Could you check a few things on this model? Use its own coordinates, in mm. A direction names the side the tool comes from. Round coordinates to 2 decimals unless told otherwise and drop trailing zeros. Write each loop counter-clockwise with the first axis right and the second up, starting at its lowest first coordinate (ties: lowest second). Pieces come first, ordered by that corner, then holes. Notation, with made-up numbers: (17, 15.25) - (66, 15.25) arc R21 cw to (66, 30.25) - close; hole circle Ø2 at (-32, -35). An arc over 180 degrees is marked (long way). Put each result on its own line as item: value.
from build123d import *

# Parameters (mm, degrees)
CHAMFER_1_SIZE      = 0.5
SKETCH_2_R          = 1.65
CUT_EXTRUDE_1_DEPTH = 10
SKETCH_3_R          = 1.65
CUT_EXTRUDE_2_DEPTH = 10


with BuildPart() as part:
    # 草图1 → 旋转1 (revolve)
    with BuildSketch(Plane(origin=(0, 0, 0), x_dir=(1, 0, 0), z_dir=(0, 1, 0)), mode=Mode.PRIVATE) as revolve_1_sk:
        Polygon((25, 8), (0, 8), (0, 2.5), (12.5, 2.5), (12.5, 4), (25, 4), align=None)
    revolve(revolve_1_sk.sketch.rotate(Axis((-10.524691358, 0, 0), (1, 0, 0)), 180), axis=Axis((-10.524691358, 0, 0), (1, 0, 0)))

    # 倒角1
    chamfer_1_edges = [part.edges().sort_by_distance(p)[0] for p in [
        (25, 0, -4),
        (12.5, 0, -2.5),
        (0, 0, -2.5),
        (0, 0, -8),
        (25, 0, -8),
    ]]
    chamfer(chamfer_1_edges, length=CHAMFER_1_SIZE)

    # 草图2 → 切除-拉伸1 (cut)
    with BuildSketch(Plane(origin=(0, 0, 0), x_dir=(1, 0, 0), z_dir=(0, 1, 0))):
        with Locations(Location((5, 0, 0), (0, 0, 270))):
            Circle(SKETCH_2_R)
        with Locations(Location((20, 0, 0), (0, 0, 270))):
            Circle(SKETCH_2_R)
    extrude(amount=-CUT_EXTRUDE_1_DEPTH, mode=Mode.SUBTRACT)

    # 草图3 → 切除-拉伸2 (cut)
    with BuildSketch(Plane.XY):
        with Locations((5, 0)):
            Circle(SKETCH_3_R)
        with Locations((20, 0)):
            Circle(SKETCH_3_R)
    extrude(amount=-CUT_EXTRUDE_2_DEPTH, mode=Mode.SUBTRACT)


solid = part.part
(1) Imagine slicing it at C-C, the plane x = 20. List the corners of the cut face in (y, z) for me.
Values found:
outline: (-7.83, -1.65) arc R8 ccw to (-1.65, -7.83) - (-1.65, -3.64) arc R4 cw to (-3.64, -1.65) - close; (-7.83, 1.65) - (-3.64, 1.65) arc R4 cw (long way) to (1.65, -3.64) - (1.65, -7.83) arc R8 ccw (long way) to start
(2) I'm going to push flat-ended pins straight in: pin 1 (6 mm diameter, centred on x = 8.5, z = 5, fed in from -Y); pin 2 (1 mm diameter, centred on x = 3.5, y = -6, fed in from -Z); pin 3 (5 mm diameter, centred on x = 7.5, z = 6.5, fed in from -Y); pin 4 (4.5 mm diameter, centred on y = 0, z = 0, fed in from -X). Where does each tip first touch, or does it pass through?
Values found:
pin 1: stops at y = -7.75
pin 2: stops at z = -5.81
pin 3: stops at y = -6.93
pin 4: passes through
(3) Please list where these lines run through material, in increasing order: probe 1 along X at (y, z) = (-5.1, 0); probe 2 along X at (y, z) = (3.5, -0.5); probe 3 along Y at (x, z) = (6, -2). Write a range as from..to.
Values found:
probe 1: x = 0..3.35, 6.65..18.35, 21.65..25
probe 2: x = 0..12.5
probe 3: y = -7.75..-1.5, 1.5..7.75
(4) For faces 1 (the face through (12.5, -3, -1)), 2 (the face through (6.524, -0.632, -4.896)), 3 (the face through (20.07, -5.79, -1.65)), which set-ups out of +Z, -Z, +X, -X, +Y, -Y let a thin tool reach every point of the face, with its end or its side?
Values found:
face 1: +X
face 2: -Z
face 3: -Y
(5) If we mould it in two halves opening along Z, with no side actions, what happens to faces 4 (the face through (12.33, 7.1, 3.69)), 5 (the face through (6.33, 2.22, 1.15)), 6 (the face through (19.785, 1.636, -5.791))? For each: pulls with the +Z half, pulls with the -Z half, needs draft (parallel to the pull), parting line crosses it, or undercut.
Values found:
face 4: parting line crosses it
face 5: undercut
face 6: needs draft
(6) Imagine slicing it at A-A, the plane y = 0. Give the number of separate pieces and of enclosed holes in the cut face, then the cut area to 3 significant figures.
Values found:
separate pieces: 4
enclosed holes: 0
area: 205 mm^2
(7) Imagine slicing it at D-D, the plane x = 23.75. List the corners of the cut face in (y, z) for me, then the cut area to 3 significant figures.
Values found:
outline: circle Ø16 at (0, 0); hole circle Ø8 at (0, 0)
area: 151 mm^2
